from build123d import *

# Parameters (mm, degrees)
SKETCH1_R           = 12
SKETCH1_R_2         = 11
BOSS_EXTRUDE1_DEPTH = 10
SKETCH2_W           = 200
SKETCH2_H           = 70
BOSS_EXTRUDE2_DEPTH = 10
CUT_EXTRUDE1_REACH  = 12
SKETCH3_R           = 11
SKETCH4_R           = 25.5
CUT_EXTRUDE2_DEPTH  = 5
SKETCH5_R           = 2.5
CUT_EXTRUDE3_DEPTH  = 40
SKETCH6_R           = 2.5
CUT_EXTRUDE4_DEPTH  = 40
FILLET1_R           = 1


with BuildPart() as part:
    # Sketch1 → Boss-Extrude1 (new body)
    with BuildSketch(Plane(origin=(0, 0, 0), x_dir=(1, 0, 0), z_dir=(0, 1, 0))):
        with Locations(Location((0, 0, 0), (0, 0, 270))):  # turned: the seam where the file's is
            Circle(SKETCH1_R)
        with Locations(Location((0, 0, 0), (0, 0, 270))):  # turned: the seam where the file's is
            Circle(SKETCH1_R_2, mode=Mode.SUBTRACT)
    extrude(amount=BOSS_EXTRUDE1_DEPTH)

    # Sketch2 → Boss-Extrude2 (add)
    with BuildSketch(Plane(origin=(0, 10, 0), x_dir=(1, 0, 0), z_dir=(0, 1, 0))):
        Rectangle(SKETCH2_W, SKETCH2_H)
    extrude(amount=BOSS_EXTRUDE2_DEPTH)

    # Sketch3 → Cut-Extrude1 (cut, up to next)
    with BuildSketch(Plane.XZ.offset(-10), mode=Mode.PRIVATE) as cut_extrude1_sk1:
        with Locations(Location((0, 0, 0), (0, 0, 270))):  # turned: the seam where the file's is
            Circle(SKETCH3_R)
    cut_extrude1_tool1 = extrude(cut_extrude1_sk1.sketch, amount=-CUT_EXTRUDE1_REACH, mode=Mode.PRIVATE) & part.part
    add(cut_extrude1_tool1.solids().sort_by_distance((0, 10, 0))[0], mode=Mode.SUBTRACT)

    # Sketch4 → Cut-Extrude2 (cut)
    with BuildSketch(Plane(origin=(0, 20, 0), x_dir=(1, 0, 0), z_dir=(0, 1, 0))):
        with Locations(Location((0, 0, 0), (0, 0, 270))):  # turned: the seam where the file's is
            Circle(SKETCH4_R)
    extrude(amount=-CUT_EXTRUDE2_DEPTH, mode=Mode.SUBTRACT)

    # Sketch5 → Cut-Extrude3 (cut)
    with BuildSketch(Plane.XY.offset(35)):
        with Locations((95, 15)):
            Circle(SKETCH5_R)
    extrude(amount=-CUT_EXTRUDE3_DEPTH, mode=Mode.SUBTRACT)

    # Sketch6 → Cut-Extrude4 (cut)
    with BuildSketch(Plane(origin=(0, 0, -35), x_dir=(-1, 0, 0), z_dir=(0, 0, -1))):
        with Locations((95, 15)):
            Circle(SKETCH6_R)
    extrude(amount=-CUT_EXTRUDE4_DEPTH, mode=Mode.SUBTRACT)

    # Fillet1
    fillet1_edges = [part.edges().sort_by_distance(p)[0] for p in [
        (100, 10, 0),
        (100, 15, 35),
        (0, 10, -35),
        (100, 15, -35),
        (-100, 10, 0),
        (-100, 15, -35),
        (0, 10, 35),
        (-100, 15, 35),
        (100, 20, 0),
        (0, 20, -35),
        (-100, 20, 0),
        (0, 20, 35),
        (92.5, 15, 35),
        (-92.5, 15, -35),
    ]]
    fillet(fillet1_edges, radius=FILLET1_R)


solid = part.part
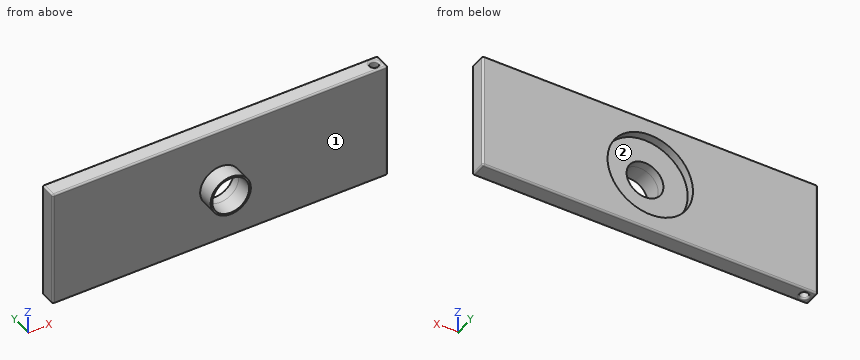
The model under review builds one solid part; all positions refer to its coordinate system, in mm. Face numbers are marked on the shaded views. Round coordinates to 2 decimals unless told otherwise and drop trailing zeros. Write each loop counter-clockwise with the first axis right and the second up, starting at its lowest first coordinate (ties: lowest second). Pieces come first, ordered by that corner, then holes. Notation, with made-up numbers: (-40, 43.5) - (-35, 43.5) arc R17 ccw to (-35, 75.5) - close; hole circle Ø7 at (-11.75, 66.25). An arc over 180 degrees is marked (long way). One line per item, written item: value. Start each with the question number.
1. The part is to be moulded in two halves that separate along Z. For the marked faces 1 and 2, say which applies: released by +Z, released by -Z, zero draft, split by the parting line, or undercut.
2. To check wall thickness, follow L1, parallel to Y at x = 95, z = 5; L2, parallel to Z at x = 0, y = 11.35; L3, parallel to Y at x = -21, z = 30. State the ranges of each line that lie inside material, in increasing order. Write a range as from..to.
3. Consider section C-C on z = 28.5. Write out the cut boundary in (x, y).
4. Consider section A-A on z = 0. Write out the cut boundary in (x, y), and give its area (3 significant figures).
5. Consider section B-B on x = 0. Write out the cut boundary in (y, z), and give its area (3 significant figures).
6. Consider section D-D on x = 95. Write out the cut boundary in (y, z), and give its area (3 significant figures).
7. Clearance check with flat-ended pins moving along their axes: P1, Ø4, axis at x = -94.5, y = 14, coming from the -Z side; P2, Ø10, axis at x = 52, z = 24, coming from the -Y side; P3, Ø15.5, axis at x = 11.5, z = 11, coming from the +Y side. State where each tip first meets the part, or that it passes through.
Checks:
1. face 1: zero draft
1. face 2: undercut
2. L1: y = 10..12.5, 17.5..20
2. L2: z = -35..-11, 11..35
2. L3: y = 10..20
3. outline: (-100, 11) arc R1 ccw to (-99, 10) - (99, 10) arc R1 ccw to (100, 11) - (100, 19) arc R1 ccw to (99, 20) - (-99, 20) arc R1 ccw to (-100, 19) - close; hole circle Ø5 at (95, 15)
4. outline: (-100, 11) arc R1 ccw to (-99, 10) - (-12, 10) - (-12, 0) - (-11, 0) - (-11, 15) - (-25.5, 15) - (-25.5, 20) - (-99, 20) arc R1 ccw to (-100, 19) - close; (11, 0) - (12, 0) - (12, 10) - (99, 10) arc R1 ccw to (100, 11) - (100, 19) arc R1 ccw to (99, 20) - (25.5, 20) - (25.5, 15) - (11, 15) - close; hole circle Ø5 at (-95, 15); hole circle Ø5 at (95, 15)
4. area: 1,610 mm^2
5. outline: (0, -12) - (10, -12) - (10, -34) arc R1 ccw to (11, -35) - (19, -35) arc R1 ccw to (20, -34) - (20, -25.5) - (15, -25.5) - (15, -11) - (0, -11) - close; (0, 11) - (15, 11) - (15, 25.5) - (20, 25.5) - (20, 34) arc R1 ccw to (19, 35) - (11, 35) arc R1 ccw to (10, 34) - (10, 12) - (0, 12) - close
5. area: 354 mm^2
6. outline: (10, -34) arc R1 ccw to (11, -35) - (19, -35) arc R1 ccw to (20, -34) - (20, 34) arc R1 ccw to (19, 35) - (18.5, 35) arc R1 ccw to (17.5, 34) - (17.5, -5) - (12.5, -5) - (12.5, 34) arc R1 ccw to (11.5, 35) - (11, 35) arc R1 ccw to (10, 34) - close
6. area: 499 mm^2
7. P1: stops at z = -34.92
7. P2: stops at y = 10
7. P3: stops at y = 15
